Autodesk Inventor part; units mm, degrees
ref_plane "YZ Plane" through (0, 0, 0) normal (1, 0, 0) x (0, 1, 0)
ref_plane "XZ Plane" through (0, 0, 0) normal (0, 1, 0) x (-1, 0, 0)
ref_plane "XY Plane" through (0, 0, 0) normal (0, 0, 1) x (1, 0, 0)
sketch "Sketch1" plane through (0, 0, 0) normal (0, 0, 1) x (1, 0, 0)
  line L0 (0, 0) -> (50.8, 0)
  line L1 (50.8, 0) -> (50.8, 50.8)
  line L2 (50.8, 50.8) -> (0, 50.8)
  line L3 (0, 50.8) -> (0, 0)
  dimension "d0" = 50.8
  dimension "d1" = 50.8
extrude "Extrusion1" add sketch "Sketch1" along normal blind 63.5
sketch "Sketch2" plane through (0, 0, 63.5) normal (0, 0, 1) x (1, 0, 0)
  line L0 (2.2085, 38.8843) -> (25.4061, 38.8843) construction
  line L1 (25.4061, 38.8843) -> (25.4061, 22.5719) construction
  line L2 (25.4061, 22.5719) -> (2.2085, 22.5719) construction
  line L3 (2.2085, 22.5719) -> (2.2085, 38.8843) construction
  spline S0 degree 2 poles (25.8795, 6.7329) (24.9533, 6.5065) (22.9361, 6.2595) (21.9275, 6.2595) knots 0 0 0 1 2 2 2
  spline S1 degree 2 poles (21.9275, 6.2595) (19.0664, 6.2595) (15.5055, 9.4499) (15.3408, 12.4139) knots 0 0 0 1 2 2 2
  spline S2 degree 2 poles (15.3408, 12.4139) (15.1144, 12.4139) (14.7233, 12.4139) (14.5586, 12.4139) knots 0 0 0 1 2 2 2
  spline S3 degree 2 poles (14.5586, 12.4139) (11.9857, 12.4139) (7.8484, 14.1635) (6.3664, 15.872) knots 0 0 0 1 2 2 2
  spline S4 degree 2 poles (6.3664, 15.872) (4.905, 17.5598) (3.3406, 22.4998) (3.3406, 25.6285) knots 0 0 0 1 2 2 2
  spline S5 degree 2 poles (3.3406, 25.6285) (3.3406, 28.8396) (4.9256, 33.6973) (6.387, 35.4263) knots 0 0 0 1 2 2 2
  spline S6 degree 2 poles (6.387, 35.4263) (7.869, 37.1347) (12.0063, 38.8843) (14.5586, 38.8843) knots 0 0 0 1 2 2 2
  spline S7 degree 2 poles (14.5586, 38.8843) (17.1521, 38.8843) (21.31, 37.0729) (22.7508, 35.4263) knots 0 0 0 1 2 2 2
  spline S8 degree 2 poles (22.7508, 35.4263) (24.1917, 33.759) (25.7972, 28.7984) (25.7972, 25.6285) knots 0 0 0 1 2 2 2
  spline S9 degree 2 poles (25.7972, 25.6285) (25.7972, 20.6885) (21.9481, 14.2665) (18.593, 13.1344) knots 0 0 0 1 2 2 2
  spline S10 degree 2 poles (18.593, 13.1344) (18.6753, 12.1875) (19.1693, 10.6643) (19.5604, 10.2321) knots 0 0 0 1 2 2 2
  spline S11 degree 2 poles (19.5604, 10.2321) (20.0338, 9.6969) (21.3306, 9.2029) (22.4833, 9.2029) knots 0 0 0 1 2 2 2
  spline S12 degree 2 poles (22.4833, 9.2029) (23.1625, 9.2029) (25.015, 9.6352) (25.4267, 9.7998) knots 0 0 0 1 2 2 2
  line L4 (25.4267, 9.7998) -> (25.8795, 9.7998)
  line L5 (25.8795, 9.7998) -> (25.8795, 6.7329)
  spline S13 degree 2 poles (22.2774, 25.6285) (22.2774, 28.1603) (21.1865, 32.0506) (20.1985, 33.3267) knots 0 0 0 1 2 2 2
  spline S14 degree 2 poles (20.1985, 33.3267) (19.1899, 34.6441) (16.3494, 35.9614) (14.5792, 35.9614) knots 0 0 0 1 2 2 2
  spline S15 degree 2 poles (14.5792, 35.9614) (12.7473, 35.9614) (9.9891, 34.6853) (8.9393, 33.3267) knots 0 0 0 1 2 2 2
  spline S16 degree 2 poles (8.9393, 33.3267) (7.9308, 32.03) (6.8604, 28.0985) (6.8604, 25.6285) knots 0 0 0 1 2 2 2
  spline S17 degree 2 poles (6.8604, 25.6285) (6.8604, 20.6267) (11.0594, 15.2956) (14.5792, 15.2956) knots 0 0 0 1 2 2 2
  spline S18 degree 2 poles (14.5792, 15.2956) (18.099, 15.2956) (22.2774, 20.6267) (22.2774, 25.6285) knots 0 0 0 1 2 2 2
  line L6 (49.1594, 12.9491) -> (44.7752, 12.9491)
  line L7 (44.7752, 12.9491) -> (36.7476, 23.0556)
  line L8 (36.7476, 23.0556) -> (32.8779, 23.0556)
  line L9 (32.8779, 23.0556) -> (32.8779, 12.9491)
  line L10 (32.8779, 12.9491) -> (29.5022, 12.9491)
  line L11 (29.5022, 12.9491) -> (29.5022, 38.3491)
  line L12 (29.5022, 38.3491) -> (36.0478, 38.3491)
  spline S19 degree 2 poles (36.0478, 38.3491) (38.2296, 38.3491) (41.1731, 37.8757) (42.511, 37.0112) knots 0 0 0 1 2 2 2
  spline S20 degree 2 poles (42.511, 37.0112) (43.8489, 36.1467) (45.3927, 33.4502) (45.3927, 31.4537) knots 0 0 0 1 2 2 2
  spline S21 degree 2 poles (45.3927, 31.4537) (45.3927, 28.6749) (42.5521, 24.9081) (40.1233, 24.0024) knots 0 0 0 1 2 2 2
  line L13 (40.1233, 24.0024) -> (49.1594, 12.9491)
  spline S22 degree 2 poles (41.8729, 31.1861) (41.8729, 32.2976) (41.0907, 34.006) (40.2674, 34.5618) knots 0 0 0 1 2 2 2
  spline S23 degree 2 poles (40.2674, 34.5618) (39.547, 35.0352) (37.6327, 35.4263) (36.233, 35.4263) knots 0 0 0 1 2 2 2
  line L14 (36.233, 35.4263) -> (32.8779, 35.4263)
  line L15 (32.8779, 35.4263) -> (32.8779, 25.8755)
  line L16 (32.8779, 25.8755) -> (35.8419, 25.8755)
  spline S24 degree 2 poles (35.8419, 25.8755) (37.3034, 25.8755) (39.6293, 26.3901) (40.432, 27.1929) knots 0 0 0 1 2 2 2
  spline S25 degree 2 poles (40.432, 27.1929) (41.1731, 27.8927) (41.8729, 29.8687) (41.8729, 31.1861) knots 0 0 0 1 2 2 2
  point P0 (0, 0)
extrude "Extrusion2" cut sketch "Sketch2" against normal blind 0.254
equation "\"d1\" = d0"
properties part number "Container 2 2 2 and half color 7"
Verification items for the finished model (mm, model axes). Round coordinates to 2 decimals unless told otherwise and drop trailing zeros. Use one line per item in the form item = value.
1. Scan line: probe 1 along Z at (x, y) = (12, 36). Record every from-to range of solid material in increasing order.
A:
probe_1 = 0 to 63.25
2. Gauge pin test, flat end, axial feed: pin 1 Ø1.5 at (y, z) = (12.5, 27.5) entering from -X. Record the tip position at first contact, or that the pin passes through.
A:
pin_1 = 0
3. Draft check along X on faces 1 (the flat face through (50.8, 25, 31)), 2 (the flat face through (26, 50.8, 31)), 3 (the flat face through (22, 19, 63.246)). Enter one of: pulls with the +X half, pulls with the -X half, needs draft (parallel to the pull), parting line crosses it, or undercut.
A:
face_1 = pulls with the +X half
face_2 = needs draft
face_3 = undercut
